Can you work these out from the model? Positions are in its coordinate system, mm. Face numbers are marked on the shaded views. A direction names the side the tool comes from. Round coordinates to 2 decimals unless told otherwise and drop trailing zeros. Loops run counter-clockwise (first coordinate to the right, second up) from the corner with the lowest first, then second, coordinate; pieces in that order, holes last.
(1) I want a section at B-B on z = 6. Give the number of separate pieces and of enclosed holes in the cut face, plus the area to 3 significant figures.
(2) Which directions (+Z, -Z, +X, -X, +Y, -Y) give clear straight access to the entire face, cutting with the end or side of a thin tool? Please do the marked faces 1, 2 and 3.
(3) I want a section at C-C on x = -15.5. Write out the boundary of the cut face in (y, z).
(4) I want a section at A-A on y = -5. Write out the boundary of the cut face in (x, z), plus the area to 3 significant figures.
(5) If I drill on line 1 along X through (y, z) = (-4.5, 7.75); line 2 along X through (y, z) = (-2, 8.5); line 3 along Z through (x, y) = (-15.5, -1.9), over which ranges is the centre line in solid material (lowest first)?
(6) I want a section at D-D on x = 0. Write out the boundary of the cut face in (y, z), plus the area to 3 significant figures.
(7) Will these pins go through, and if not, where does the flat tip stop? pin 1 Ø2.5 at (x, z) = (15.5, 6) entering from +Y; pin 2 Ø1.6 at (y, z) = (-0.5, 5) entering from +X; pin 3 Ø2.5 at (x, z) = (14.5, 4.5) entering from +Y; pin 4 Ø7 at (x, z) = (15.5, 6) entering from -Y.
(8) Thinking about a two-plate mould opening in X: for the marked faces 4, 5 and 6, which applies, released by +X, released by -X, zero draft, split by the parting line, or undercut?
from build123d import *
from OCP.BRepFilletAPI import BRepFilletAPI_MakeChamfer

# Parameters (mm, degrees)
BOSS_EXTRUDE1_DEPTH = 12
SKETCH4_R           = 2.1
CUT_EXTRUDE1_DEPTH  = 27.646669586
SKETCH5_W           = 17.126081539
SKETCH5_H           = 14.483771816
CUT_EXTRUDE2_DEPTH  = 31.50036885
FILLET2_R           = 0.75
SKETCH7_R           = 4.25
CUT_EXTRUDE4_DEPTH  = 0.6
CHAMFER1_SIZE       = 2
CHAMFER1_SIZE2      = 1.678199262


with BuildPart() as part:
    # Sketch1 → Boss-Extrude1 (new body)
    with BuildSketch(Plane.XY):
        with BuildLine():
            Line((-11.15, 0), (-11.15, -1.5))
            Line((-11.15, -1.5), (-20.15, -1.5))
            Line((-20.15, -1.5), (-20.15, -8.5))
            Line((-20.15, -8.5), (-6.15, -8.5))
            Line((-6.15, -8.5), (-6.15, 0))
            ThreePointArc((-6.15, 0), (0, 6.15), (6.15, 0))
            Line((6.15, 0), (6.15, -8.5))
            Line((6.15, -8.5), (20.15, -8.5))
            Line((20.15, -8.5), (20.15, -1.5))
            Line((20.15, -1.5), (11.15, -1.5))
            Line((11.15, -1.5), (11.15, 0))
            ThreePointArc((11.15, 0), (0, 11.15), (-11.15, 0))
        make_face()
    extrude(amount=BOSS_EXTRUDE1_DEPTH)

    # Sketch4 → Cut-Extrude1 (cut, through all)
    with BuildSketch(Plane(origin=(0, -1.5, 0), x_dir=(1, 0, 0), z_dir=(0, 1, 0))):
        with Locations(Location((-15.5, -6, 0), (0, 0, 180))):
            Circle(SKETCH4_R)
        with Locations(Location((15.5, -6, 0), (0, 0, 180))):
            Circle(SKETCH4_R)
    extrude(amount=-CUT_EXTRUDE1_DEPTH, mode=Mode.SUBTRACT)

    # Sketch5 → Cut-Extrude2 (cut, through all)
    with BuildSketch(Plane(origin=(0, 11, 0), x_dir=(1, 0, 0), z_dir=(0, 1, 0))):
        with Locations((0.195726647, -5.794276843)):
            Rectangle(SKETCH5_W, SKETCH5_H)
    extrude(amount=CUT_EXTRUDE2_DEPTH, mode=Mode.SUBTRACT)

    # Fillet2
    fillet2_edges = [part.edges().sort_by_distance(p)[0] for p in [
        (20.15, -5, 0),
        (6.15, -4.25, 0),
        (0, 6.15, 0),
        (-6.15, -4.25, 0),
        (-20.15, -5, 0),
        (-20.15, -5, 12),
        (-6.15, -4.25, 12),
        (0, 6.15, 12),
        (6.15, -4.25, 12),
        (20.15, -5, 12),
    ]]
    fillet(fillet2_edges, radius=FILLET2_R)

    # Sketch7 → Cut-Extrude4 (cut)
    with BuildSketch(Plane(origin=(0, -1.5, 0), x_dir=(1, 0, 0), z_dir=(0, 1, 0))):
        with Locations(Location((-15.5, -6, 0), (0, 0, 180))):
            Circle(SKETCH7_R)
        with Locations(Location((15.5, -6, 0), (0, 0, 180))):
            Circle(SKETCH7_R)
    extrude(amount=-CUT_EXTRUDE4_DEPTH, mode=Mode.SUBTRACT)

    # Chamfer1: one chamfer whose edges measure the first distance from different faces: ONE call of the kernel's chamfer builder (chamfer() names one face for all edges)
    chamfer1_edges_1 = [part.edges().sort_by_distance(p)[0] for p in [
        (-13.4, -2.1, 6),
    ]]
    chamfer1_side_1 = [part.faces().sort_by_distance(p)[0] for p in [
        (-13.4, -5.3, 6),
    ]]
    chamfer1_edges_2 = [part.edges().sort_by_distance(p)[0] for p in [
        (17.6, -2.1, 6),
    ]]
    chamfer1_side_2 = [part.faces().sort_by_distance(p)[0] for p in [
        (17.6, -5.3, 6),
    ]]
    chamfer1 = BRepFilletAPI_MakeChamfer(part.part.solid().wrapped)
    for e in chamfer1_edges_1:
        chamfer1.Add(CHAMFER1_SIZE, CHAMFER1_SIZE2, e.wrapped, chamfer1_side_1[0].wrapped)  # the first distance lies on this face
    for e in chamfer1_edges_2:
        chamfer1.Add(CHAMFER1_SIZE, CHAMFER1_SIZE2, e.wrapped, chamfer1_side_2[0].wrapped)  # the first distance lies on this face
    add(Compound.cast(chamfer1.Shape()), mode=Mode.REPLACE)


solid = part.part
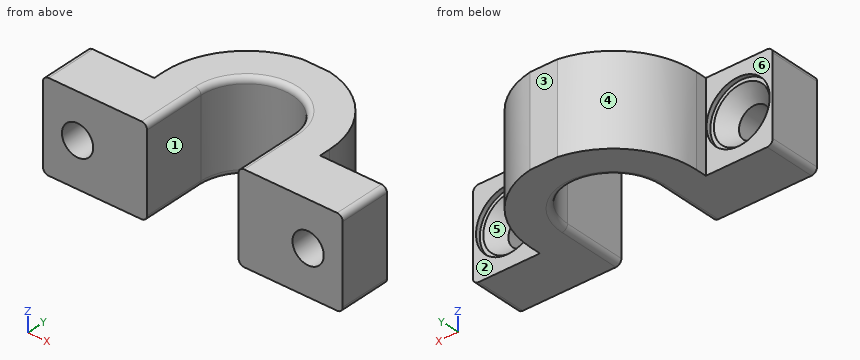
Filled sheet:
1. separate pieces: 3
1. enclosed holes: 0
1. area: 276 mm2
2. face 1: +Z, -Z, -Y
2. face 2: +Z, -Z, +X, +Y
2. face 3: +Z, -Z, +X, -X, +Y
3. outline: (-8.5, 0) - (-1.5, 0) - (-1.5, 1.75) - (-2.1, 1.75) - (-2.1, 2.22) - (-4.1, 3.9) - (-8.5, 3.9) - close; (-8.5, 8.1) - (-4.1, 8.1) - (-2.1, 9.78) - (-2.1, 10.25) - (-1.5, 10.25) - (-1.5, 12) - (-8.5, 12) - close
4. outline: (-20.15, 0.75) arc R0.75 ccw to (-19.4, 0) - (-6.9, 0) arc R0.75 ccw to (-6.15, 0.75) - (-6.15, 11.25) arc R0.75 ccw to (-6.9, 12) - (-19.4, 12) arc R0.75 ccw to (-20.15, 11.25) - close; (6.15, 0.75) arc R0.75 ccw to (6.9, 0) - (19.4, 0) arc R0.75 ccw to (20.15, 0.75) - (20.15, 11.25) arc R0.75 ccw to (19.4, 12) - (6.9, 12) arc R0.75 ccw to (6.15, 11.25) - close; hole circle Ø4.2 at (-15.5, 6); hole circle Ø4.2 at (15.5, 6)
4. area: 307 mm2
5. line 1: x = -20.15 to -16.66, -14.34 to -6.15, 6.15 to 14.34, 16.66 to 20.15
5. line 2: x = -20.15 to -18.94, -12.06 to -6.15, 6.15 to 12.06, 18.94 to 20.15
5. line 3: z = 0 to 1.75, 10.25 to 12
6. outline: (6.15, 0.75) arc R0.75 ccw to (6.9, 0) - (11, 0) - (11, 12) - (6.9, 12) arc R0.75 ccw to (6.15, 11.25) - close
6. area: 58.0 mm2
7. pin 1: passes through
7. pin 2: stops at x = 11.15
7. pin 3: stops at y = -2.96
7. pin 4: stops at y = -8.5
8. face 4: released by -X
8. face 5: undercut
8. face 6: zero draft
